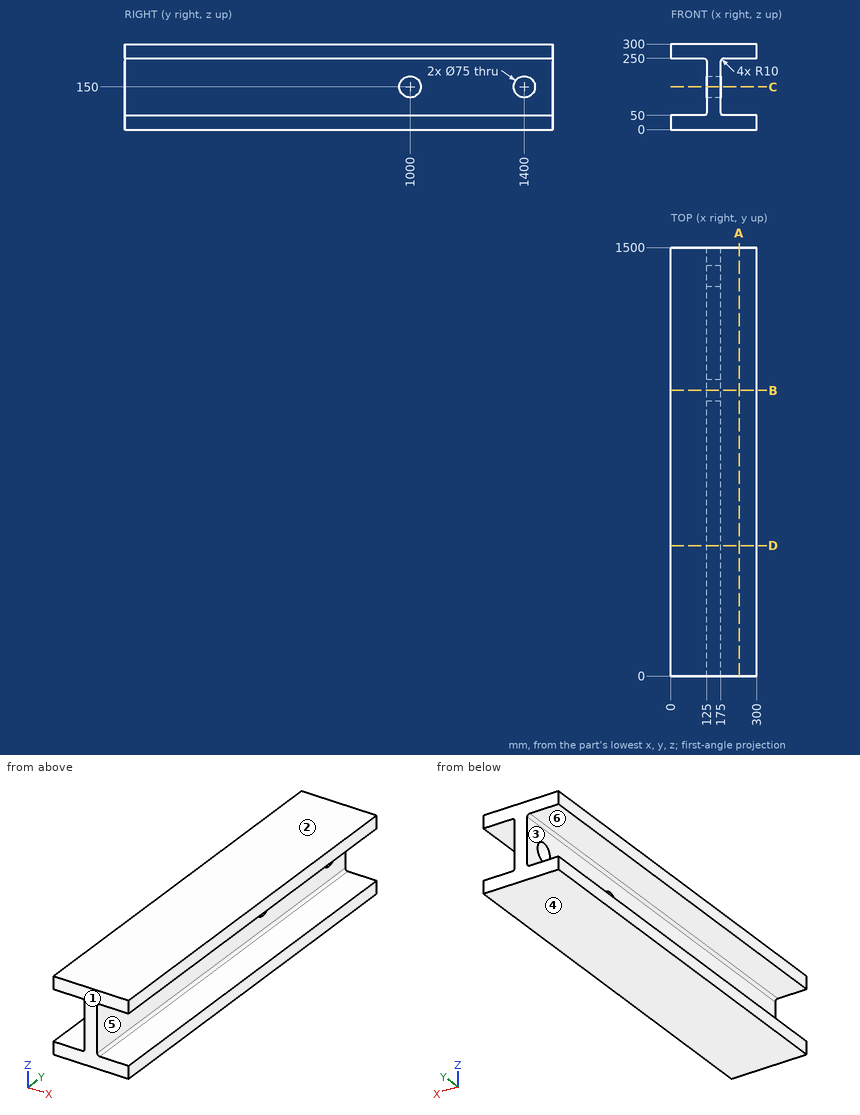
Here's the drawing with two shaded views (mm, measured from the low corner). I have some questions. A direction names the side the tool comes from. Coordinates: 2 decimals unless noted, no trailing zeros. Loops run counter-clockwise (first coordinate to the right, second up) from the corner with the lowest first, then second, coordinate; pieces in that order, holes last. Notation, with made-up numbers: M -28.75,-3 L 16.25,-3 A27 cw 16.25,35 Z; hole C 75,-16 d6. An arc over 180 degrees is marked long. Put each result on its own line as item: value. Start each with the question number.
(1) Imagine slicing it at B-B on y = 1000. List the corners of the cut face in (x, z) for me.
(2) We'd pull the mould along Z, two halves only. Please class the marked faces 1, 2 and 3: +Z half, -Z half, draft (parallel to the pull), parting line (faces both ways), or undercut.
(3) Imagine slicing it at D-D on y = 457. List the corners of the cut face in (x, z) for me, and give its area (3 significant figures).
(4) I need wall thicknesses on probe 1 along Y at (x, z) = (151.5, 150); probe 2 along Z at (x, y) = (214.5, 62.5); probe 3 along X at (y, z) = (539, 92.5). Which ranges of each line are inside material? Lowest first, please.
(5) Imagine slicing it at A-A on x = 239.5. List the corners of the cut face in (y, z) for me, and give its area (3 significant figures).
(6) Which directions (+Z, -Z, +X, -X, +Y, -Y) give clear straight access to the entire face, cutting with the end or side of a thin tool? Please do the marked faces 4, 5 and 6.
(7) Imagine slicing it at C-C on z = 150. List the corners of the cut face in (x, y) for me.
(8) Will these pins go through, and if not, where does the flat tip stop? pin 1 Ø6 at (y, z) = (778, 115.5) entering from +X; pin 2 Ø1 at (y, z) = (816, 106.5) entering from -X.
Worked answers:
1. outline: M 0,0 L 300,0 L 300,50 L 185,50 A10 cw 175,60 L 175,112.5 L 125,112.5 L 125,60 A10 cw 115,50 L 0,50 Z; M 0,250 L 115,250 A10 cw 125,240 L 125,187.5 L 175,187.5 L 175,240 A10 cw 185,250 L 300,250 L 300,300 L 0,300 Z
2. face 1: draft
2. face 2: +Z half
2. face 3: undercut
3. outline: M 0,0 L 300,0 L 300,50 L 185,50 A10 cw 175,60 L 175,240 A10 cw 185,250 L 300,250 L 300,300 L 0,300 L 0,250 L 115,250 A10 cw 125,240 L 125,60 A10 cw 115,50 L 0,50 Z
3. area: 40,100 mm2
4. probe 1: y = 0 to 962.5, 1037.5 to 1362.5, 1437.5 to 1500
4. probe 2: z = 0 to 50, 250 to 300
4. probe 3: x = 125 to 175
5. outline: M 0,0 L 1500,0 L 1500,50 L 0,50 Z; M 0,250 L 1500,250 L 1500,300 L 0,300 Z
5. area: 150,000 mm2
6. face 4: -Z, +X, -X, +Y, -Y
6. face 5: +X, +Y, -Y
6. face 6: -X, +Y, -Y
7. outline: M 125,0 L 175,0 L 175,962.5 L 125,962.5 Z; M 125,1037.5 L 175,1037.5 L 175,1362.5 L 125,1362.5 Z; M 125,1437.5 L 175,1437.5 L 175,1500 L 125,1500 Z
8. pin 1: stops at x = 175
8. pin 2: stops at x = 125
